The drawing under review shows one solid part. Ordinate dimensions are in mm from its lowest x, y, z. A direction names the side the tool comes from. Round coordinates to 2 decimals unless told otherwise and drop trailing zeros. Write each loop counter-clockwise with the first axis right and the second up, starting at its lowest first coordinate (ties: lowest second). Pieces come first, ordered by that corner, then holes.
Item 1: Draft analysis for pull direction Y (two halves, no side actions). For the marked faces 1, 2 and 3, state which applies: +Y half, -Y half, draft (parallel to the pull), parting line (faces both ways), or undercut.
Item 2: Add section D-D (z = 35). Give the boundary of the cut face in (x, y), plus the area to 4 significant figures.
Item 3: Clearance check with a flat-ended pin moving along its axis: pin 1 Ø3.5 at (x, z) = (5, 35) entering from +Y. State where the tip first meets the part, or that it passes through.
Item 4: Add section B-B (y = 8). Give the boundary of the cut face in (x, z).
Item 5: To check wall thickness, follow L1, parallel to Z at x = 5, y = 9.1; L2, parallel to X at y = 2.5, z = 7. State the ranges of each line that lie inside material, in increasing order.
Item 6: Machinability: for the marked faces 4 and 5, which of the approach directions +Z, -Z, +X, -X, +Y, -Y give a long, thin tool a straight path to every point of the face, cutting with its end or side? Answer none if there is none.
Item 7: Add section C-C (z = 11). Give the boundary of the cut face in (x, y), plus the area to 3 significant figures.
Item 8: Add section A-A (x = 5). Give the boundary of the cut face in (y, z).
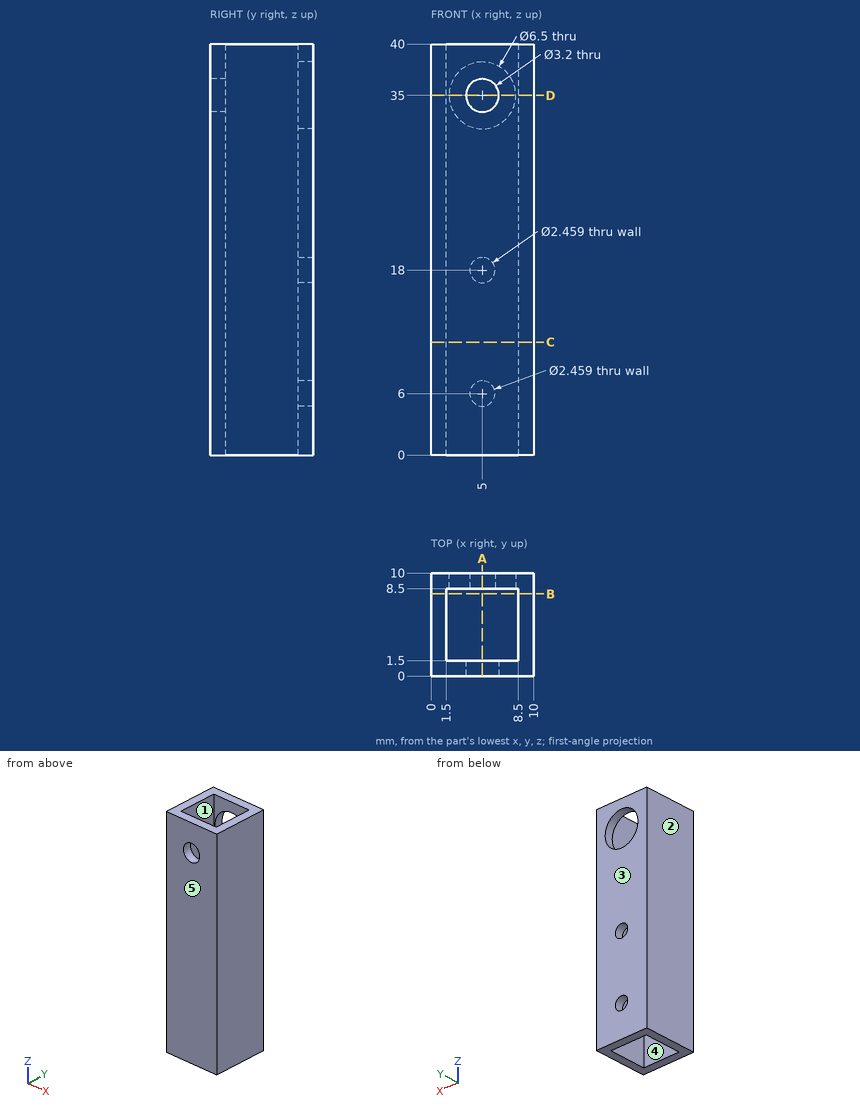
Numbers:
1. face 1: undercut
1. face 2: draft
1. face 3: +Y half
2. outline: (0, 0) - (3.4, 0) - (3.4, 1.5) - (1.5, 1.5) - (1.5, 8.5) - (1.75, 8.5) - (1.75, 10) - (0, 10) - close; (6.6, 0) - (10, 0) - (10, 10) - (8.25, 10) - (8.25, 8.5) - (8.5, 8.5) - (8.5, 1.5) - (6.6, 1.5) - close
2. area: 36.45 mm2
3. pin 1: stops at y = 1.5
4. outline: (0, 0) - (1.5, 0) - (1.5, 40) - (0, 40) - close; (8.5, 0) - (10, 0) - (10, 40) - (8.5, 40) - close
5. L1: z = 0 to 4.77, 7.23 to 16.77, 19.23 to 31.75, 38.25 to 40
5. L2: x = 0 to 1.5, 8.5 to 10
6. face 4: +Z, -Z
6. face 5: +Z, -Z, +X, -X, -Y
7. outline: (0, 0) - (10, 0) - (10, 10) - (0, 10) - close; hole (1.5, 1.5) - (8.5, 1.5) - (8.5, 8.5) - (1.5, 8.5) - close
7. area: 51.0 mm2
8. outline: (0, 0) - (1.5, 0) - (1.5, 33.4) - (0, 33.4) - close; (0, 36.6) - (1.5, 36.6) - (1.5, 40) - (0, 40) - close; (8.5, 0) - (10, 0) - (10, 4.77) - (8.5, 4.77) - close; (8.5, 7.23) - (10, 7.23) - (10, 16.77) - (8.5, 16.77) - close; (8.5, 19.23) - (10, 19.23) - (10, 31.75) - (8.5, 31.75) - close; (8.5, 38.25) - (10, 38.25) - (10, 40) - (8.5, 40) - close
